The drawing under review shows one solid part. Ordinate dimensions are in mm from its lowest x, y, z. A direction names the side the tool comes from. Give positions to 0.01 mm unless a question says otherwise; leave off trailing zeros. Order: outer loops, then holes, each group sorted by start corner. A loop starts at its lowest first (then second) coordinate and runs counter-clockwise, first axis right, second up. Notation, with made-up numbers: (12, 79) - (58, 79) arc R19 cw to (58, 98) - close; hole circle Ø7 at (67, 32.25). An arc over 180 degrees is marked (long way). Use CSV: the item, a comma, the result in double quotes. Start each with the question number.
1. Take a section at C-C, the plane z = 12.25. State the section outline as (x, y) points.
2. To check wall thickness, follow line 1 (X direction, y = 2.8, z = 1.25); line 2 (Z direction, x = 2.6, y = 5.25) (1 decimal); line 3 (Z direction, x = 3.05, y = 3.25). State the ranges of each line that lie inside material, in increasing order. Write a range as [from, to].
3. For pin 1 (1.3 mm diameter, centred on y = 3.5, z = 18.5, fed in from -X); pin 2 (0.6 mm diameter, centred on y = 4, z = 18, fed in from +X) (1 decimal); pin 3 (0.6 mm diameter, centred on x = 2.5, z = 18.5, fed in from +Y), all flat-tipped, find the tip position at first contact; note any pin that passes through.
4. Machinability: for the marked faces 1 and 2, which of the approach directions +Z, -Z, +X, -X, +Y, -Y give a long, thin tool a straight path to every point of the face, cutting with its end or side? Answer none if there is none.
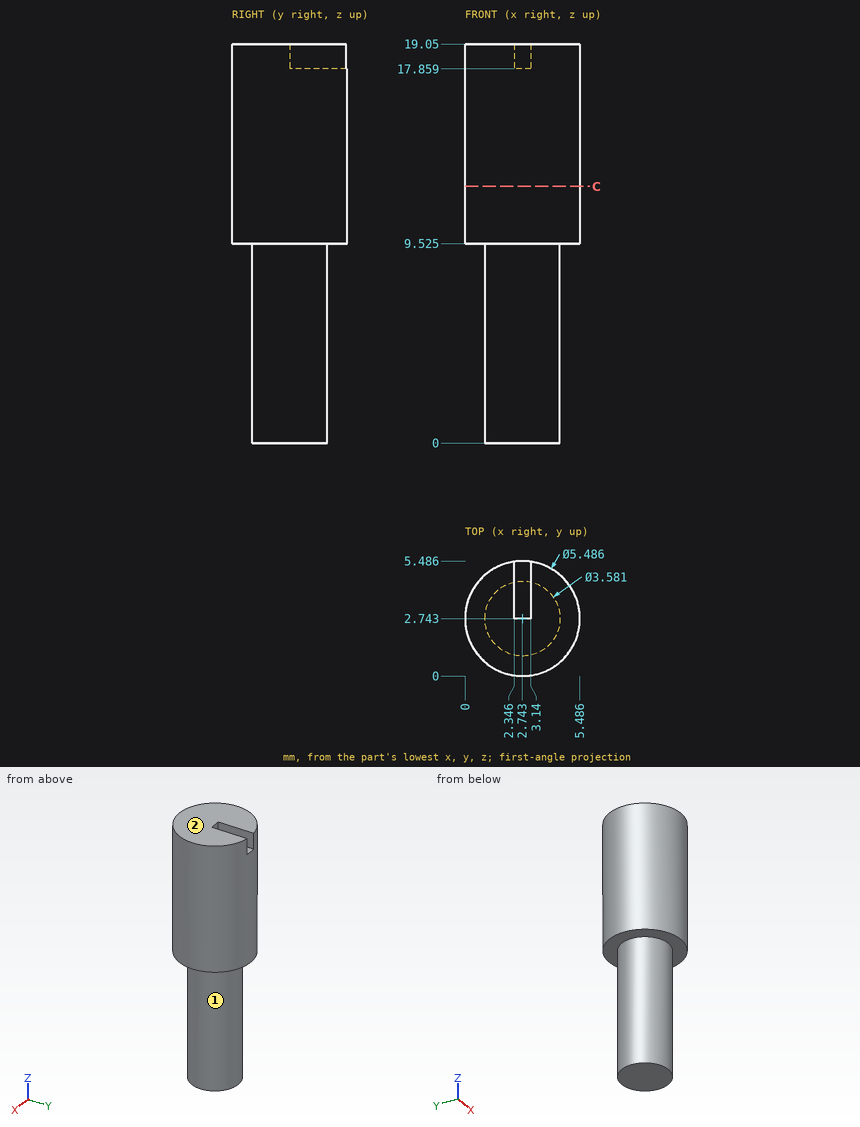
Determined:
1,outline,"circle Ø5.49 at (2.74, 2.74)"
2,line 1,"x = [0.95, 4.53]"
2,line 2,"z = [9.5, 17.9]"
2,line 3,"z = [0, 17.86]"
3,pin 1,"stops at x = 0"
3,pin 2,"stops at x = 5.3"
3,pin 3,"stops at y = 5.46"
4,face 1,"-Z"
4,face 2,"+Z, +X, -X, +Y, -Y"
